Verification items for this drawing (mm, ordinates from the low corner). Give positions to 0.01 mm unless a question says otherwise; leave off trailing zeros. Loops run counter-clockwise (first coordinate to the right, second up) from the corner with the lowest first, then second, coordinate; pieces in that order, holes last. Notation, with made-up numbers: M 49,69 L 108,69 A7 ccw 108,80 Z; hole C 49,17.25 d5. An arc over 180 degrees is marked long. Write each question's results on one line, items separated by ' | '. Start each with the question number.
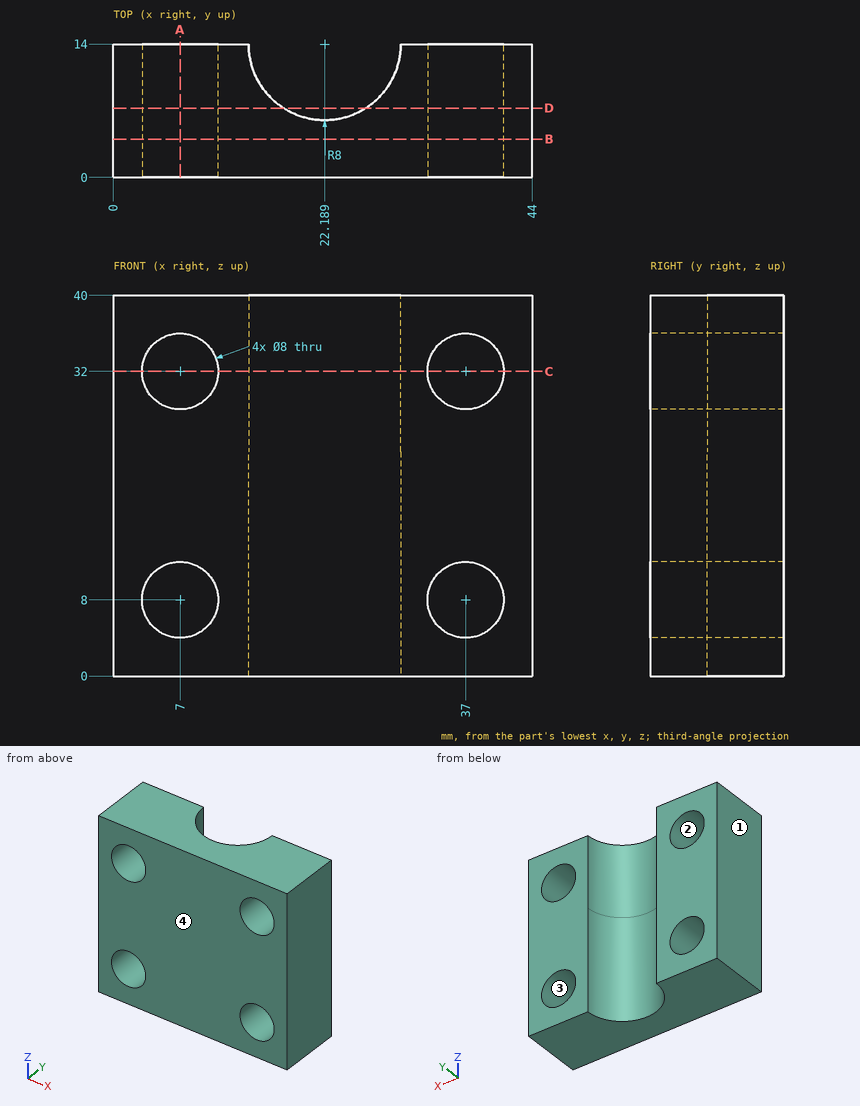
1. Section check A-A, the plane x = 7. Record the boundary of the cut face in (y, z), plus the area to 3 significant figures.
2. Section check C-C, the plane z = 32. Record the boundary of the cut face in (x, y).
3. Section check B-B, the plane y = 4. Record the boundary of the cut face in (x, z).
4. Release check for a two-part mould opening along X. For the marked faces 1, 2, 3 and 4 record: released by +X, released by -X, zero draft, split by the parting line, or undercut.
5. Section check D-D, the plane y = 7.25. Record the boundary of the cut face in (x, z) (3 decimals).
6. Thickness scan on probe 1 along X at (y, z) = (4, 32); probe 2 along Z at (x, y) = (7, 8.5); probe 3 along X at (y, z) = (10.25, 31.5). Record the ranges inside material, lowest first.
Filled sheet:
1) outline: M 0,0 L 14,0 L 14,4 L 0,4 Z; M 0,12 L 14,12 L 14,28 L 0,28 Z; M 0,36 L 14,36 L 14,40 L 0,40 Z | area: 336 mm2
2) outline: M 0,0 L 3,0 L 3,14 L 0,14 Z; M 11,0 L 33,0 L 33,14 L 30.19,14 A8 cw 14.19,14 L 11,14 Z; M 41,0 L 44,0 L 44,14 L 41,14 Z
3) outline: M 0,0 L 44,0 L 44,40 L 0,40 Z; hole C 7,8 d8; hole C 7,32 d8; hole C 37,8 d8; hole C 37,32 d8
4) face 1: released by -X | face 2: undercut | face 3: undercut | face 4: zero draft
5) outline: M 0,0 L 17.895,0 L 17.895,40 L 0,40 Z; M 26.483,0 L 44,0 L 44,40 L 26.483,40 Z; hole C 7,8 d8; hole C 7,32 d8; hole C 37,8 d8; hole C 37,32 d8
6) probe 1: 0 to 3, 11 to 33, 41 to 44 | probe 2: 0 to 4, 12 to 28, 36 to 40 | probe 3: 0 to 3.03, 10.97 to 15.12, 29.26 to 33.03, 40.97 to 44
